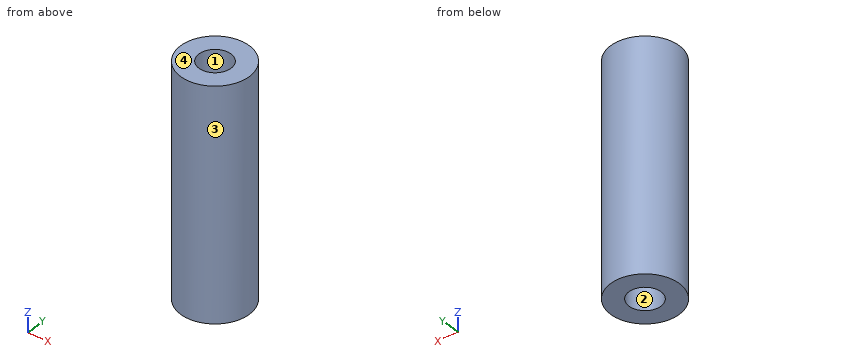
Autodesk Inventor part; units mm, degrees
ref_plane "YZ Plane" through (0, 0, 0) normal (1, 0, 0) x (0, 1, 0)
ref_plane "XZ Plane" through (0, 0, 0) normal (0, 1, 0) x (-1, 0, 0)
ref_plane "XY Plane" through (0, 0, 0) normal (0, 0, 1) x (1, 0, 0)
sketch "スケッチ1" plane through (0, 0, 0) normal (0, 0, 1) x (1, 0, 0)
  circle A0 centre (0, 0) radius 3
  dimension "d0" = 6
extrude "押し出し1" add sketch "スケッチ1" along normal blind 20
sketch "スケッチ2" plane through (0, 0, 20) normal (0, 0, 1) x (1, 0, 0)
  circle A0 centre (0, 0) radius 1.4
  dimension "d3" = 2.8
extrude "押し出し2" cut sketch "スケッチ2" against normal blind 6
sketch "スケッチ3" plane through (0, 0, 0) normal (0, 0, -1) x (-1, 0, 0)
  circle A0 centre (0, 0) radius 1.4
  circle A1 centre (0, 0) radius 1.4
extrude "押し出し3" cut sketch "スケッチ3" against normal blind 6
properties part number "34mm" material "アルミニウム 6061"
Input: part model. Units: mm. Frame: model coordinates. Face numbers are marked on the shaded views. Coordinates: 2 decimals unless noted, no trailing zeros. Loops run counter-clockwise (first coordinate to the right, second up) from the corner with the lowest first, then second, coordinate; pieces in that order, holes last.
Q1. Cut plane D-D (z = 8.5). Output: boundary loops of the cut face in (x, y), then the cut area to 3 significant figures.
Q2. Cut plane C-C (z = 17.5). Output: boundary loops of the cut face in (x, y).
Q3. Draft query along Y for the marked faces 1, 2, 3 and 4. Return one class per face: +Y half, -Y half, draft (parallel to the pull), parting line (faces both ways), or undercut.
Q4. Material intervals for line 1 (Y direction, x = 0, z = 15.95); line 2 (Z direction, x = -0.8, y = 1.1); line 3 (Y direction, x = 1.25, z = 5.75), sorted ascending.
Q5. Cut plane A-A (y = 0). Output: boundary loops of the cut face in (x, z), then the cut area to 3 significant figures.
Q6. Contact query for flat-ended pins moving along their axis: pin 1 (2.5 mm diameter, centred on x = 0, y = 0, fed in from +Z); pin 2 (1.5 mm diameter, centred on x = 1, z = 11.5, fed in from +Y); pin 3 (1.4 mm diameter, centred on x = 0, y = 0.5, fed in from -Z). Output: stop coordinate, or through.
Working result:
1. outline: circle Ø6 at (0, 0)
1. area: 28.3 mm2
2. outline: circle Ø6 at (0, 0); hole circle Ø2.8 at (0, 0)
3. face 1: undercut
3. face 2: undercut
3. face 3: parting line
3. face 4: draft
4. line 1: y = -3 to -1.4, 1.4 to 3
4. line 2: z = 6 to 14
4. line 3: y = -2.73 to -0.63, 0.63 to 2.73
5. outline: (-3, 0) - (-1.4, 0) - (-1.4, 6) - (1.4, 6) - (1.4, 0) - (3, 0) - (3, 20) - (1.4, 20) - (1.4, 14) - (-1.4, 14) - (-1.4, 20) - (-3, 20) - close
5. area: 86.4 mm2
6. pin 1: stops at z = 14
6. pin 2: stops at y = 2.99
6. pin 3: stops at z = 6
